Can you work these out from the model? Positions are in its coordinate system, mm. Give positions to 0.01 mm unless a question says otherwise; leave off trailing zeros. Loops run counter-clockwise (first coordinate to the right, second up) from the corner with the lowest first, then second, coordinate; pieces in that order, holes last. Notation, with made-up numbers: (31.5, 18.25) - (60.5, 18.25) arc R8 cw to (60.5, 24.25) - close; hole circle Ø5 at (-3.75, -25). An arc over 180 degrees is marked (long way). Write item = value, one per line.
from build123d import *

# Parameters (mm, degrees)
SKETCH1_W           = 12.7
SKETCH1_H           = 139.7
BOSS_EXTRUDE1_DEPTH = 12.7
CHAMFER1_SIZE       = 9.525
SKETCH2_R           = 1.905
CUT_EXTRUDE1_DEPTH  = 141.849813631
SKETCH3_R           = 1.905
CUT_EXTRUDE2_DEPTH  = 141.849813631
FILLET1_R           = 6.35


with BuildPart() as part:
    # Sketch1 → Boss-Extrude1 (new body)
    with BuildSketch(Plane.XY):
        with Locations((6.35, 69.85)):
            Rectangle(SKETCH1_W, SKETCH1_H)
    extrude(amount=BOSS_EXTRUDE1_DEPTH)

    # Chamfer1
    chamfer1_edges = [part.edges().sort_by_distance(p)[0] for p in [
        (0, 69.85, 0),
    ]]
    chamfer(chamfer1_edges, length=CHAMFER1_SIZE)

    # Sketch2 → Cut-Extrude1 (cut, through all)
    with BuildSketch(Plane.XY.offset(12.7)):
        with Locations((6.35, 133.35)):
            Circle(SKETCH2_R)
        with Locations((6.35, 6.35)):
            Circle(SKETCH2_R)
    extrude(amount=-CUT_EXTRUDE1_DEPTH, mode=Mode.SUBTRACT)

    # Sketch3 → Cut-Extrude2 (cut, through all)
    with BuildSketch(Plane(origin=(12.7, 0, 0), x_dir=(0, 0, -1), z_dir=(1, 0, 0))):
        with Locations((-6.35, 127)):
            Circle(SKETCH3_R)
        with Locations((-6.35, 12.7)):
            Circle(SKETCH3_R)
    extrude(amount=-CUT_EXTRUDE2_DEPTH, mode=Mode.SUBTRACT)

    # Fillet1
    # the kernel refuses this fillet: 6.35 mm, written as the material it takes off along each edge
    with BuildSketch(Plane(origin=(28.575, 139.7, 0), x_dir=(0, -1, 0), z_dir=(-1, 0, 0)), Plane(origin=(0, 139.7, -6.35), x_dir=(0, -1, 0), z_dir=(0, 0, 1)), Plane(origin=(0, 0, -6.35), x_dir=(1, 0, 0), z_dir=(0, 0, 1))) as fillet1_piece_1:
        with BuildLine():
            CenterArc((FILLET1_R, FILLET1_R), FILLET1_R, 180, 90)
            Line((0, FILLET1_R), (0, 0))
            Line((0, 0), (FILLET1_R, 0))
        make_face()
    extrude(amount=34.925, mode=Mode.SUBTRACT)
    with BuildSketch(Plane(origin=(-6.35, 0, 0), x_dir=(0, 0, 1), z_dir=(1, 0, 0))) as fillet1_piece_2:
        with BuildLine():
            CenterArc((FILLET1_R, -FILLET1_R), FILLET1_R, 90, 90)
            Line((0, -FILLET1_R), (0, 0))
            Line((0, 0), (FILLET1_R, 0))
        make_face()
    extrude(amount=34.925, mode=Mode.SUBTRACT)


solid = part.part
Q1. For pin 1 (3 mm diameter, centred on x = 6.35, y = 133.35, fed in from -Z); pin 2 (3 mm diameter, centred on x = 3, z = 9.5, fed in from +Y); pin 3 (5 mm diameter, centred on x = 6.35, y = 6.35, fed in from -Z) (3 decimals); pin 4 (6 mm diameter, centred on y = 12.7, z = 6.35, fed in from -X) (3 decimals), each with a flat end and sliding along its axis, tell me the tip position at first contact or that it passes through.
Output:
pin_1 = through
pin_2 = 139.42
pin_3 = 0.675
pin_4 = 0.175
Q2. Imagine slicing it at B-B, the plane x = 2.75. Write out the boundary of the cut face in (y, z) (3 decimals), then the cut area to 3 significant figures.
Output:
outline = (1.119, 6.775) - (10.843, 6.775) arc R1.905 cw to (14.557, 6.775) - (125.143, 6.775) arc R1.905 cw to (128.857, 6.775) - (138.581, 6.775) - (138.581, 12.7) - (1.119, 12.7) - close
area = 806 mm2
Q3. I need wall thicknesses on L1, parallel to Y at x = 6.35, z = 9 (3 decimals); L2, parallel to Y at x = 9, z = 6.35 (3 decimals); L3, parallel to Y at x = 6, z = 7. Which ranges of each line are inside material? Lowest first, please.
Output:
L1 = 0 to 4.445, 8.255 to 131.445, 135.255 to 139.7
L2 = 0 to 10.795, 14.605 to 125.095, 128.905 to 139.7
L3 = 0.01 to 4.48, 8.22 to 10.91, 14.49 to 125.21, 128.79 to 131.48, 135.22 to 139.69
Q4. Imagine slicing it at A-A, the plane y = 12.7. Write out the boundary of the cut face in (x, z) (3 decimals).
Output:
outline = (0, 9.525) - (1.27, 8.255) - (12.7, 8.255) - (12.7, 12.7) - (0, 12.7) - close; (5.08, 4.445) - (9.525, 0) - (12.7, 0) - (12.7, 4.445) - close
Q5. We'd pull the mould along Y, two halves only. Please class faces 1 (the flat face through (12.7, 69, 6)), 2 (the cylindrical face through (8.167, 133.922, 8.335)), 3 (the flat face through (9, 139.7, 9)): released by +Y, released by -Y, zero draft, split by the parting line, or undercut.
Output:
face_1 = zero draft
face_2 = undercut
face_3 = released by +Y
